from build123d import *

# Parameters (mm, degrees)
SKETCH_5_R                   = 22.5
EXTRUDE_2_DEPTH              = 10
HOLE_WIZARD_M3_1_D           = 3.4
HOLE_WIZARD_M3_1_CBORE_D     = 6.5
HOLE_WIZARD_M3_1_CBORE_DEPTH = 3
SKETCH_12_W                  = 25
SKETCH_12_H                  = 40
CUT_EXTRUDE_1_DEPTH          = 3
EXTRUDE_3_DEPTH              = 1
SKETCH_14_R                  = 1.75
CUT_EXTRUDE_2_DEPTH          = 3
MIRROR_2_COPY_1_DEPTH        = 1
MIRROR_2_COPY_2_SKETCH_R     = 1.75
MIRROR_2_COPY_2_DEPTH        = 3
SKETCH_16_R                  = 7.5
CUT_EXTRUDE_3_DEPTH          = 11
EXTRUDE_4_DEPTH              = 3


with BuildPart() as part:
    # ｽｹｯﾁ5 → ﾎﾞｽ - 押し出し2 (new body)
    with BuildSketch(Plane.XY):
        Circle(SKETCH_5_R)
    extrude(amount=EXTRUDE_2_DEPTH)

    # M3 穴付きねじ用座ぐり穴1 (through all)
    with Locations(Plane.XY.offset(10)):
        with Locations((19, 0), (-19, 0)):
            CounterBoreHole(HOLE_WIZARD_M3_1_D / 2, HOLE_WIZARD_M3_1_CBORE_D / 2, HOLE_WIZARD_M3_1_CBORE_DEPTH)

    # ｽｹｯﾁ12 → ｶｯﾄ - 押し出し1 (cut)
    with BuildSketch(Plane(origin=(0, 0, 0), x_dir=(-1, 0, 0), z_dir=(0, 0, -1))):
        with Locations((0, -2.5)):
            Rectangle(SKETCH_12_W, SKETCH_12_H)
    extrude(amount=-CUT_EXTRUDE_1_DEPTH, mode=Mode.SUBTRACT)

    # ｽｹｯﾁ13 → ﾎﾞｽ - 押し出し3 (add)
    with BuildSketch(Plane(origin=(0, 0, 3), x_dir=(-1, 0, 0), z_dir=(0, 0, -1))):
        with BuildLine():
            Line((-12.5, 3), (-9, 3))
            ThreePointArc((-9, 3), (-6.5, 5.5), (-9, 8))
            Line((-9, 8), (-12.5, 8))
            Line((-12.5, 8), (-12.5, 3))
        make_face()
    extrude_3 = extrude(amount=EXTRUDE_3_DEPTH)

    # ｽｹｯﾁ14 → ｶｯﾄ - 押し出し2 (cut)
    with BuildSketch(Plane(origin=(0, 0, 2), x_dir=(-1, 0, 0), z_dir=(0, 0, -1))):
        with Locations((-9, 5.5)):
            Circle(SKETCH_14_R)
    cut_extrude_2 = extrude(amount=-CUT_EXTRUDE_2_DEPTH, mode=Mode.SUBTRACT)

    # ﾐﾗｰ1: ﾎﾞｽ - 押し出し3, ｶｯﾄ - 押し出し2 across plane
    add(extrude_3.mirror(Plane(origin=(0, 0, 0), x_dir=(0, 0, 1), z_dir=(1, 0, 0))))
    add(cut_extrude_2.mirror(Plane(origin=(0, 0, 0), x_dir=(0, 0, 1), z_dir=(1, 0, 0))), mode=Mode.SUBTRACT)

    # ﾐﾗｰ2: ﾎﾞｽ - 押し出し3, ｶｯﾄ - 押し出し2 across plane
    add(extrude_3.mirror(Plane.ZX))
    add(cut_extrude_2.mirror(Plane.ZX), mode=Mode.SUBTRACT)

    # ﾐﾗｰ2 copy 1 sketch → ﾐﾗｰ2 copy 1 (add)
    with BuildSketch(Plane(origin=(0, 0, 3), x_dir=(1, 0, 0), z_dir=(0, 0, -1))):
        with BuildLine():
            Line((-12.5, 3), (-9, 3))
            ThreePointArc((-9, 3), (-6.5, 5.5), (-9, 8))
            Line((-9, 8), (-12.5, 8))
            Line((-12.5, 8), (-12.5, 3))
        make_face()
    extrude(amount=MIRROR_2_COPY_1_DEPTH)

    # ﾐﾗｰ2 copy 2 sketch → ﾐﾗｰ2 copy 2 (cut)
    with BuildSketch(Plane(origin=(0, 0, 2), x_dir=(1, 0, 0), z_dir=(0, 0, -1))):
        with Locations((-9, 5.5)):
            Circle(MIRROR_2_COPY_2_SKETCH_R)
    extrude(amount=-MIRROR_2_COPY_2_DEPTH, mode=Mode.SUBTRACT)

    # ｽｹｯﾁ16 → ｶｯﾄ - 押し出し3 (cut, through all)
    with BuildSketch(Plane.XY.offset(10)):
        Circle(SKETCH_16_R)
    extrude(amount=-CUT_EXTRUDE_3_DEPTH, mode=Mode.SUBTRACT)

    # ｽｹｯﾁ17 → ﾎﾞｽ - 押し出し4 (add)
    with BuildSketch(Plane(origin=(0, 0, 0), x_dir=(-1, 0, 0), z_dir=(0, 0, -1))):
        with BuildLine():
            ThreePointArc((22.5, 0), (19.843134833, -10.606601718), (12.5, -18.708286934))
            Line((12.5, -18.708286934), (12.5, -19.899748742))
            ThreePointArc((12.5, -19.899748742), (20.566963801, -11.368817001), (23.5, 0))
            ThreePointArc((23.5, 0), (-11.368817001, 20.566963801), (-12.5, -19.899748742))
            Line((-12.5, -19.899748742), (-12.5, -18.708286934))
            ThreePointArc((-12.5, -18.708286934), (-10.606601718, 19.843134833), (22.5, 0))
        make_face()
    extrude(amount=-EXTRUDE_4_DEPTH)


solid = part.part
Part model, mm, in its own coordinate system. A direction names the side the tool comes from. Round coordinates to 2 decimals unless told otherwise and drop trailing zeros. Order: outer loops, then holes, each group sorted by start corner. A loop starts at its lowest first (then second) coordinate and runs counter-clockwise, first axis right, second up. Notation, with made-up numbers: (88, 86) -> (120, 86) arc R15 cw to (120, 96) -> close; hole circle Ø10 at (51.25, 80.25). An arc over 180 degrees is marked (long way). Put each result on its own line as item: value.
Q1. Band-saw the part on A-A (x = 0). Give the cut face in (y, z).
From the geometry:
outline: (-22.5, 3) -> (-7.5, 3) -> (-7.5, 10) -> (-22.5, 10) -> close; (7.5, 3) -> (17.5, 3) -> (17.5, 0) -> (23.5, 0) -> (23.5, 3) -> (22.5, 3) -> (22.5, 10) -> (7.5, 10) -> close
Q2. Tool access for faces 5 (the face through (-10.7, -8, 2.5)), 6 (the face through (-9, 6, 5)), 7 (the face through (20.784, -8.618, 6.451)): list every direction of +Z, -Z, +X, -X, +Y, -Y with a clear straight run to the whole face (end or side of a thin tool).
From the geometry:
face 5: -Z, -Y
face 6: -Z
face 7: +Z
Q3. Pin check, flat tips, straight feed: pin 1 Ø2.5 at (x, y) = (10, -4.5) entering from -Z; pin 2 Ø1 at (y, z) = (12, 7.5) entering from +X; pin 3 Ø0.5 at (x, z) = (11, 2.5) entering from -Y; pin 4 Ø6 at (x, y) = (12, 0) entering from -Z. Stop position of each tip, or through.
From the geometry:
pin 1: stops at z = 2
pin 2: stops at x = 19.34
pin 3: stops at y = -8
pin 4: stops at z = 0
Q4. Pull direction Y, two halves, no side cores. Call faces 1 (the face through (10.7, -8, 2.5)), 2 (the face through (10.8, 3, 2.5)), 3 (the face through (10.8, -3, 2.5)), 4 (the face through (0, 23, 3)): pulls with the +Y half, pulls with the -Y half, needs draft (parallel to the pull), parting line crosses it, or undercut.
From the geometry:
face 1: pulls with the -Y half
face 2: undercut
face 3: undercut
face 4: needs draft
Q5. Band-saw the part on C-C (y = 5.5). Give the cut face in (x, z).
From the geometry:
outline: (-22.85, 0) -> (-12.5, 0) -> (-12.5, 2) -> (-10.75, 2) -> (-10.75, 5) -> (-7.25, 5) -> (-7.25, 2) -> (-6.5, 2) -> (-6.5, 3) -> (-5.1, 3) -> (-5.1, 10) -> (-21.82, 10) -> (-21.82, 3) -> (-22.85, 3) -> close; (5.1, 3) -> (6.5, 3) -> (6.5, 2) -> (7.25, 2) -> (7.25, 5) -> (10.75, 5) -> (10.75, 2) -> (12.5, 2) -> (12.5, 0) -> (22.85, 0) -> (22.85, 3) -> (21.82, 3) -> (21.82, 10) -> (5.1, 10) -> close
Q6. Wall check: line 1 (X direction, y = -5.5, z = 2.8); line 2 (X direction, y = -1, z = 1); line 3 (Z direction, x = -6.5, y = -13). Give the ranges that are in metal, low to high. Write a range as [from, to].
From the geometry:
line 1: x = [-22.85, -10.75], [-7.25, -6.5], [6.5, 7.25], [10.75, 22.85]
line 2: x = [-23.48, -20.37], [-17.63, -12.5], [12.5, 17.63], [20.37, 23.48]
line 3: z = [3, 10]
Q7. Band-saw the part on D-D (y = 19). Give the cut face in (x, z), and give its area (3 significant figures).
From the geometry:
outline: (-13.83, 0) -> (13.83, 0) -> (13.83, 3) -> (12.05, 3) -> (12.05, 10) -> (-12.05, 10) -> (-12.05, 3) -> (-13.83, 3) -> close
area: 252 mm2
Q8. Band-saw the part on B-B (z = 0.75). Give the cut face in (x, y), and give its area (3 significant figures).
From the geometry:
outline: (-12.5, -19.9) -> (-12.5, 17.5) -> (12.5, 17.5) -> (12.5, -19.9) arc R23.5 ccw (long way) to start; hole circle Ø3.4 at (-19, 0); hole circle Ø3.4 at (19, 0)
area: 721 mm2
